The model under review builds one solid part; all positions refer to its coordinate system, in mm. Face numbers are marked on the shaded views. A direction names the side the tool comes from. Round coordinates to 2 decimals unless told otherwise and drop trailing zeros. Order: outer loops, then holes, each group sorted by start corner. A loop starts at its lowest first (then second) coordinate and runs counter-clockwise, first axis right, second up.
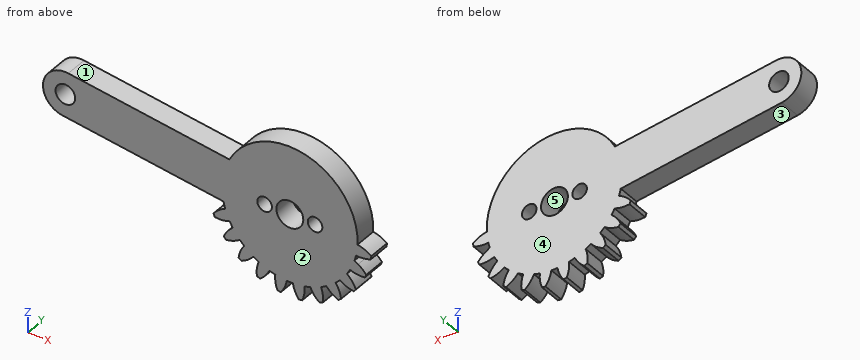
```python
from build123d import *

# Parameters (mm, degrees)
SKETCH1_R           = 1.75
SKETCH1_R_2         = 2.4
SKETCH1_R_3         = 1.3
BOSS_EXTRUDE1_DEPTH = 4


with BuildPart() as part:
    # Sketch1 → Boss-Extrude1 (new body)
    with BuildSketch(Plane(origin=(0, 4, 0), x_dir=(1, 0, 0), z_dir=(0, 1, 0))):
        with BuildLine():
            Line((1.43808022, 3.600125745), (2.081641936, 4))
            ThreePointArc((2.081641936, 4), (2.861028333, 4.588201733), (3.521749436, 5.30713988))
            ThreePointArc((3.521749436, 5.30713988), (3.405395609, 5.596745198), (3.282888305, 5.883801663))
            ThreePointArc((3.282888305, 5.883801663), (1.93527598, 5.894040025), (0.627094961, 5.57027124))
            ThreePointArc((0.627094961, 5.57027124), (0.366286148, 6.046375), (0.084372603, 6.510293938))
            ThreePointArc((0.084372603, 6.510293938), (1.018855105, 7.48132754), (1.683794586, 8.65351323))
            ThreePointArc((1.683794586, 8.65351323), (1.496450048, 8.903135899), (1.303821399, 9.148703928))
            ThreePointArc((1.303821399, 9.148703928), (-0.000522033, 8.809805691), (-1.180330337, 8.158486898))
            ThreePointArc((-1.180330337, 8.158486898), (-1.555477026, 8.550865528), (-1.947855656, 8.926012217))
            ThreePointArc((-1.947855656, 8.926012217), (-1.296536862, 10.105820521), (-0.957638625, 11.410163953))
            ThreePointArc((-0.957638625, 11.410163953), (-1.203206655, 11.602792602), (-1.452829324, 11.79013714))
            ThreePointArc((-1.452829324, 11.79013714), (-2.625015014, 11.125197659), (-3.596048616, 10.190715157))
            ThreePointArc((-3.596048616, 10.190715157), (-4.059967554, 10.472628702), (-4.536071314, 10.733437515))
            ThreePointArc((-4.536071314, 10.733437515), (-4.212302529, 12.041618533), (-4.222540891, 13.389230859))
            ThreePointArc((-4.222540891, 13.389230859), (-4.509597355, 13.511738163), (-4.799202674, 13.62809199))
            ThreePointArc((-4.799202674, 13.62809199), (-5.759348103, 12.682425791), (-6.455432668, 11.528463019))
            ThreePointArc((-6.455432668, 11.528463019), (-6.976508546, 11.680699536), (-7.503891752, 11.809396783))
            ThreePointArc((-7.503891752, 11.809396783), (-7.529737283, 13.156800143), (-7.888414517, 14.455843809))
            ThreePointArc((-7.888414517, 14.455843809), (-8.197396993, 14.499881098), (-8.507248835, 14.537314892))
            ThreePointArc((-8.507248835, 14.537314892), (-9.18992168, 13.375367565), (-9.563620196, 12.080565177))
            ThreePointArc((-9.563620196, 12.080565177), (-10.106342554, 12.09275), (-10.649064912, 12.080565177))
            ThreePointArc((-10.649064912, 12.080565177), (-11.022763428, 13.375367565), (-11.705436272, 14.537314892))
            ThreePointArc((-11.705436272, 14.537314892), (-12.015288115, 14.499881098), (-12.324270591, 14.455843809))
            ThreePointArc((-12.324270591, 14.455843809), (-12.682947825, 13.156800143), (-12.708793355, 11.809396783))
            ThreePointArc((-12.708793355, 11.809396783), (-13.236176561, 11.680699536), (-13.757252439, 11.528463019))
            ThreePointArc((-13.757252439, 11.528463019), (-14.453337005, 12.682425791), (-15.413482434, 13.62809199))
            ThreePointArc((-15.413482434, 13.62809199), (-15.703087752, 13.511738163), (-15.990144217, 13.389230859))
            ThreePointArc((-15.990144217, 13.389230859), (-16.000382579, 12.041618533), (-15.676613793, 10.733437515))
            ThreePointArc((-15.676613793, 10.733437515), (-16.152717554, 10.472628702), (-16.616636492, 10.190715157))
            ThreePointArc((-16.616636492, 10.190715157), (-17.587670094, 11.125197659), (-18.759855783, 11.79013714))
            ThreePointArc((-18.759855783, 11.79013714), (-19.009478453, 11.602792602), (-19.255046482, 11.410163953))
            ThreePointArc((-19.255046482, 11.410163953), (-18.916148245, 10.105820521), (-18.264829452, 8.926012217))
            ThreePointArc((-18.264829452, 8.926012217), (-18.657208082, 8.550865528), (-19.032354771, 8.158486898))
            ThreePointArc((-19.032354771, 8.158486898), (-20.212163074, 8.809805691), (-21.516506507, 9.148703928))
            ThreePointArc((-21.516506507, 9.148703928), (-21.709135156, 8.903135899), (-21.896479694, 8.65351323))
            ThreePointArc((-21.896479694, 8.65351323), (-21.231540213, 7.48132754), (-20.297057711, 6.510293938))
            ThreePointArc((-20.297057711, 6.510293938), (-20.578971255, 6.046375), (-20.839780068, 5.57027124))
            ThreePointArc((-20.839780068, 5.57027124), (-22.147961087, 5.894040025), (-23.495573413, 5.883801663))
            ThreePointArc((-23.495573413, 5.883801663), (-23.618080717, 5.596745198), (-23.734434544, 5.30713988))
            ThreePointArc((-23.734434544, 5.30713988), (-22.788768345, 4.346994451), (-21.634805572, 3.650909885))
            ThreePointArc((-21.634805572, 3.650909885), (-21.803584999, 3.067429176), (-21.942853375, 2.47620963))
            Line((-21.942853375, 2.47620963), (-50.694754355, -1.309049944))
            ThreePointArc((-50.694754355, -1.309049944), (-54.138429032, -5.796934159), (-49.650544818, -9.240608835))
            Line((-49.650544818, -9.240608835), (-20.898643838, -5.455349261))
            ThreePointArc((-20.898643838, -5.455349261), (-7.038913378, -11.697242445), (1.974222624, 0.542722358))
            ThreePointArc((1.974222624, 0.542722358), (3.269025011, 0.916420874), (4.430972339, 1.599093719))
            ThreePointArc((4.430972339, 1.599093719), (4.393538544, 1.908945561), (4.349501255, 2.217928037))
            ThreePointArc((4.349501255, 2.217928037), (3.050457589, 2.576605271), (1.70305423, 2.602450802))
            ThreePointArc((1.70305423, 2.602450802), (1.581217534, 3.104116905), (1.43808022, 3.600125745))
        make_face()
        with Locations(Location((-50.172649586, -5.27482939, 0), (0, 0, 90))):
            Circle(SKETCH1_R, mode=Mode.SUBTRACT)
        with Locations(Location((-10.106342554, 0, 0), (0, 0, 90))):
            Circle(SKETCH1_R_2, mode=Mode.SUBTRACT)
        with Locations(Location((-5.606342554, 0, 0), (0, 0, 90))):
            Circle(SKETCH1_R_3, mode=Mode.SUBTRACT)
        with Locations(Location((-14.606342554, 0, 0), (0, 0, 90))):
            Circle(SKETCH1_R_3, mode=Mode.SUBTRACT)
    extrude(amount=-BOSS_EXTRUDE1_DEPTH)


solid = part.part
```
(1) Insertion check: pin 1 (3 mm diameter, centred on x = -50.17, z = 5.27, fed in from -Y). The pin has a flat end and moves straight along its axis. Give the tip position at first contact, or say it passes through.
Data:
pin 1: passes through
(2) For the marked faces 1 and 2, list the 3-axis set-ups (+Z, -Z, +X, -X, +Y, -Y) from which the entire face can be reached by the end or side of a thin tool; tool diameter is ignored.
Data:
face 1: +Z, +Y, -Y
face 2: +Z, -Z, +X, -X, -Y
(3) Consider section D-D (z = -4.75). Write out the cut boundary in (x, y), and give its area (3 significant figures).
Data:
outline: (-23.24, 0) - (3.03, 0) - (3.03, 4) - (-23.24, 4) - close
area: 105 mm2
(4) Consider section C-C (x = -38). Write out the cut boundary in (y, z), and give its area (3 significant figures).
Data:
outline: (0, -0.36) - (4, -0.36) - (4, 7.71) - (0, 7.71) - close
area: 32.3 mm2
(5) Consider section B-B (y = 2.4). State how many separate pieces and enclosed holes the cut face has, and give its area (3 significant figures).
Data:
separate pieces: 1
enclosed holes: 4
area: 719 mm2
(6) Draft analysis for pull direction X (two halves, no side actions). For the marked faces 3, 4 and 5, state which applies: pulls with the +X half, pulls with the -X half, needs draft (parallel to the pull), parting line crosses it, or undercut.
Data:
face 3: pulls with the -X half
face 4: needs draft
face 5: undercut
(7) To check wall thickness, follow probe 1 along X at (y, z) = (3.5, -13) (3 decimals); probe 2 along Z at (x, y) = (-14.5, 2.55); probe 3 along X at (y, z) = (2.75, -12). State the ranges of each line that lie inside material, in increasing order.
Data:
probe 1: x = -16.028 to -14.724, -12.703 to -10.878, -9.335 to -7.509, -5.488 to -4.185
probe 2: z = -12.74 to -1.3, 1.3 to 11.27
probe 3: x = -16 to -13.99, -12.73 to -7.49, -6.22 to -4.22
(8) Consider section A-A (z = 0). Write out the cut boundary in (x, y), and give its area (3 significant figures).
Data:
outline: (-40.75, 0) - (-15.91, 0) - (-15.91, 4) - (-40.75, 4) - close; (-13.31, 0) - (-12.51, 0) - (-12.51, 4) - (-13.31, 4) - close; (-7.71, 0) - (-6.91, 0) - (-6.91, 4) - (-7.71, 4) - close; (-4.31, 0) - (1.99, 0) - (1.99, 4) - (-4.31, 4) - close
area: 131 mm2
